from build123d import *

# Parameters (mm, degrees)
ESBO_O1_W                                      = 130
ESBO_O1_H                                      = 22
RESSALTO_EXTRUS_O1_DEPTH                       = 95
CORTE_EXTRUS_O2_REACH                          = 24
CORTE_EXTRUS_O3_DEPTH                          = 1
CORTE_EXTRUS_O3_DEPTH_BACK                     = 66
BROCA_DE_ROSQUEAR_DE_CANO_PARA_TARRAXA_D_D     = 6.579997
BROCA_DE_ROSQUEAR_DE_CANO_PARA_TARRAXA_D_DEPTH = 10
BROCA_DE_ROSQUEAR_DE_CANO_PARA_TARRAXA_D_TIP   = 1.976830535
BROCA_DE_ROSQUEAR_DE_CANO_PARA_TARRA_2_D       = 6.579997
BROCA_DE_ROSQUEAR_DE_CANO_PARA_TARRA_2_DEPTH   = 10
BROCA_DE_ROSQUEAR_DE_CANO_PARA_TARRA_2_TIP     = 1.976830535
FILETE2_R                                      = 5
ESBO_O16_W                                     = 47.75
ESBO_O16_H                                     = 2
CORTE_EXTRUS_O6_DEPTH                          = 40
FILETE3_R                                      = 3


with BuildPart() as part:
    # Esboço1 → Ressalto-extrusão1 (new body)
    with BuildSketch(Plane.XY):
        Rectangle(ESBO_O1_W, ESBO_O1_H)
    extrude(amount=RESSALTO_EXTRUS_O1_DEPTH)

    # Esboço2 → Corte-extrusão2 (cut, up to next)
    with BuildSketch(Plane(origin=(0, 11, 0), x_dir=(1, 0, 0), z_dir=(0, 1, 0)), mode=Mode.PRIVATE) as corte_extrus_o2_sk1:
        with BuildLine():
            Line((17.25, 0), (-65, 0))
            Line((-65, 0), (-65, -95))
            Line((-65, -95), (0, -95))
            ThreePointArc((0, -95), (26.860074256, -72.440999729), (40.2, -40))
            Line((40.2, -40), (17.25, 0))
        make_face()
    corte_extrus_o2_tool1 = extrude(corte_extrus_o2_sk1.sketch, amount=-CORTE_EXTRUS_O2_REACH, mode=Mode.PRIVATE) & part.part
    add(corte_extrus_o2_tool1.solids().sort_by_distance((-18.119573, 11, 46.581056))[0], mode=Mode.SUBTRACT)

    # Esboço3 → Corte-extrusão3 (cut, two sides)
    with BuildSketch(Plane(origin=(65, 0, 0), x_dir=(0, 0, -1), z_dir=(1, 0, 0))) as corte_extrus_o3_sk:
        Polygon((200.195338438, 55.253706392), (0, 11), (-95, -10), (-295.195338438, -54.253706392), (-383.702751221, 346.136970485), (111.687925655, 455.644383268), align=None)
    extrude(amount=CORTE_EXTRUS_O3_DEPTH, mode=Mode.SUBTRACT)
    extrude(corte_extrus_o3_sk.sketch, amount=-CORTE_EXTRUS_O3_DEPTH_BACK, mode=Mode.SUBTRACT)

    # Broca de rosquear de cano para tarraxa d
    with Locations(Plane(origin=(65, 0, 0), x_dir=(0, 0, -1), z_dir=(1, 0, 0))):
        with Locations((-20, -2.945)):
            Hole(BROCA_DE_ROSQUEAR_DE_CANO_PARA_TARRAXA_D_D / 2, depth=BROCA_DE_ROSQUEAR_DE_CANO_PARA_TARRAXA_D_DEPTH)
            with Locations((0, 0, -(BROCA_DE_ROSQUEAR_DE_CANO_PARA_TARRAXA_D_DEPTH + BROCA_DE_ROSQUEAR_DE_CANO_PARA_TARRAXA_D_TIP / 2))):  # 118° drill point
                Cone(0, BROCA_DE_ROSQUEAR_DE_CANO_PARA_TARRAXA_D_D / 2, BROCA_DE_ROSQUEAR_DE_CANO_PARA_TARRAXA_D_TIP, mode=Mode.SUBTRACT)

    # Broca de rosquear de cano para tarra 2
    with Locations(Plane(origin=(12.977837756, 0, -7.446034412), x_dir=(0.497656085, 0, 0.867374441), z_dir=(-0.867374441, 0, 0.497656085))):
        with Locations((28.584567474, -2.945)):
            Hole(BROCA_DE_ROSQUEAR_DE_CANO_PARA_TARRA_2_D / 2, depth=BROCA_DE_ROSQUEAR_DE_CANO_PARA_TARRA_2_DEPTH)
            with Locations((0, 0, -(BROCA_DE_ROSQUEAR_DE_CANO_PARA_TARRA_2_DEPTH + BROCA_DE_ROSQUEAR_DE_CANO_PARA_TARRA_2_TIP / 2))):  # 118° drill point
                Cone(0, BROCA_DE_ROSQUEAR_DE_CANO_PARA_TARRA_2_D / 2, BROCA_DE_ROSQUEAR_DE_CANO_PARA_TARRA_2_TIP, mode=Mode.SUBTRACT)

    # Filete2
    filete2_edges = [part.edges().sort_by_distance(p)[0] for p in [
        (65, -10.5, 95),
    ]]
    fillet(filete2_edges, radius=FILETE2_R)

    # Esboço16 → Corte-extrusão6 (cut)
    with BuildSketch(Plane(origin=(0, 0, 0), x_dir=(-1, 0, 0), z_dir=(0, 0, -1))):
        with Locations((-41.125, -10)):
            Rectangle(ESBO_O16_W, ESBO_O16_H)
    extrude(amount=-CORTE_EXTRUS_O6_DEPTH, mode=Mode.SUBTRACT)

    # Filete3
    filete3_edges = [part.edges().sort_by_distance(p)[0] for p in [
        (40.2, -3.421052632, 40),
    ]]
    fillet(filete3_edges, radius=FILETE3_R)


solid = part.part
Here's how the part is built. I have some questions about the finished solid (model axes, mm). A direction names the side the tool comes from. Round coordinates to 2 decimals unless told otherwise and drop trailing zeros. Write each loop counter-clockwise with the first axis right and the second up, starting at its lowest first coordinate (ties: lowest second). Pieces come first, ordered by that corner, then holes.
1. Will these pins go through, and if not, where does the flat tip stop? pin 1 Ø6 at (y, z) = (-2.945, 20) entering from +X; pin 2 Ø10 at (y, z) = (1, 67.5) entering from -X; pin 3 Ø3 at (y, z) = (-5, 41.5) entering from -X.
2. Suppose I cut it at B-B (z = 29). List the corners of the cut face in (x, y) for me.
3. If we mould it in two halves opening along Z, with no side actions, what happens to faces 1 (the cylindrical face through (59.93, -1.96, 23.14)), 2 (the flat face through (41, 1, 0)), 3 (the cylindrical face through (64, -10, 93))? For each: released by +Z, released by -Z, zero draft, split by the parting line, or undercut.
4. For faces 4 (the conical face through (37.08, -2.56, 11.19)), 5 (the cylindrical face through (30.906, -7.32, 66.279)), 6 (the flat face through (47, -9, 20)), which set-ups out of +Z, -Z, +X, -X, +Y, -Y let a thin tool reach every point of the face, with its end or its side?
5. Suppose I cut it at A-A (x = 45). List the corners of the cut face in (y, z) for me, and give its area (3 significant figures).
6. Suppose I cut it at C-C (y = 9.75). List the corners of the cut face in (x, z) for me, and give its area (3 significant figures).
7. I need wall thicknesses on L1, parallel to Y at x = 61, z = 20 (3 decimals); L2, parallel to Y at x = 43.5, z = 47.5; L3, parallel to X at y = -8.5, z = 78. Which ranges of each line are inside material? Lowest first, please.
Answer sheet:
1. pin 1: stops at x = 54.83
1. pin 2: stops at x = 29.98
1. pin 3: stops at x = 39.69
2. outline: (33.89, -9) - (65, -9) - (65, 4.59) - (33.89, 4.59) - close
3. face 1: undercut
3. face 2: released by -Z
3. face 3: released by +Z
4. face 4: none
4. face 5: -X, +Y, -Y
4. face 6: -Z, +X, -X, -Y
5. outline: (-11, 40) - (-9, 40) - (-9, 0) - (11, 0) - (-10, 95) - (-11, 95) - close
5. area: 1,010 mm2
6. outline: (17.25, 0) - (65, 0) - (65, 5.65) - (20.49, 5.65) - close
6. area: 261 mm2
7. L1: y = -9 to -6.235, 0.345 to 6.579
7. L2: y = -11 to 0.5
7. L3: x = 22.37 to 65
